Autodesk Inventor part; units mm, degrees
ref_plane "YZ Plane" through (0, 0, 0) normal (1, 0, 0) x (0, 1, 0)
ref_plane "XZ Plane" through (0, 0, 0) normal (0, 1, 0) x (-1, 0, 0)
ref_plane "XY Plane" through (0, 0, 0) normal (0, 0, 1) x (1, 0, 0)
sketch "Sketch1" plane through (0, 0, 0) normal (0, 1, 0) x (-1, 0, 0)
  circle A0 centre (0, 0) radius 3.975
  circle A1 centre (0, 0) radius 5.965
  dimension "d0" = 7.95
  dimension "d1" = 11.93
extrude "Extrusion1" add sketch "Sketch1" along normal blind 7
sketch "Sketch2" plane through (0, 7, 0) normal (0, 1, 0) x (1, 0, 0)
  circle A0 centre (0, 0) radius 5.965
  circle A1 centre (0, 0) radius 11
  dimension "d4" = 22
extrude "Extrusion2" add sketch "Sketch2" against normal up to surface (7 mm away)
sketch "Sketch3" plane through (0, 0, 0) normal (0, -1, 0) x (1, 0, 0)
  circle A0 centre (0, 0) radius 5.96
  circle A1 centre (0, 0) radius 9.725
  dimension "d7" = 11.92
  dimension "d8" = 19.45
extrude "Extrusion3" cut sketch "Sketch3" against normal blind 0.25
sketch "Sketch4" plane through (0, 7, 0) normal (0, 1, 0) x (1, 0, 0)
  circle A0 centre (0, 0) radius 5.96
  circle A1 centre (0, 0) radius 9.725
  circle A2 centre (0, 0) radius 5.96
  circle A3 centre (0, 0) radius 9.725
extrude "Extrusion4" cut sketch "Sketch4" against normal blind 0.25
properties part number "bearing_1"
For this review, take the finished solid that the model builds, in its own axes (mm). A direction names the side the tool comes from. Coordinates: 2 decimals unless noted, no trailing zeros. Loops run counter-clockwise (first coordinate to the right, second up) from the corner with the lowest first, then second, coordinate; pieces in that order, holes last. Notation, with made-up numbers: (20, -3.5) - (53, -3.5) arc R21 ccw to (53, 22.5) - close; hole circle Ø2 at (31.25, 71). An arc over 180 degrees is marked (long way). Use a Markdown table: item, result. Add a question column.
Item 1: We need section A-A (z = 0). Give the boundary of the cut face in (x, y) (3 decimals), and give its area (3 significant figures).
Item 2: Tool access review of faces 1 (the face through (-4.5, 0.25, -4.2)), 2 (the face through (1.4, 0, -3.9)): name each direction out of +Z, -Z, +X, -X, +Y, -Y from which nothing blocks a thin tool from reaching the whole face with its end or side.
Item 3: Mouldability with a two-part tool opening along X and no side actions: class faces 3 (the face through (1.4, 7, -3.9)), 4 (the face through (-4.5, 6.75, 4.2)), 5 (the face through (-2.38, 3.55, 10.74)) as pulls with the +X half, pulls with the -X half, needs draft (parallel to the pull), parting line crosses it, or undercut.
Item 4: We need section D-D (z = 8). Give the boundary of the cut face in (x, y).
Item 5: For line 1 (Z direction, x = 0, y = 0.1) (3 decimals); line 2 (Z direction, x = -0.75, y = 3); line 3 (Y direction, x = 2.75, z = 6), list the stretches that pass through material, from the lowest coordinate up.
Item 6: We need section B-B (x = 0). Give the boundary of the cut face in (y, z) (3 decimals).
Item 7: Insertion check: pin 1 Ø1.5 at (x, y) = (8.5, 5) entering from +Z; pin 2 Ø7 at (x, z) = (0, 0) entering from +Y. Each pin has a flat end and moves straight along its axis. Give the tip position at first contact, or say it passes through.
Item 8: We need section C-C (y = 5.25). Give the boundary of the cut face in (x, z) (3 decimals).
Results list:
| question | item | result |
|---|---|---|
| 1 | outline | (-11, 0) - (-9.725, 0) - (-9.725, 0.25) - (-5.96, 0.25) - (-5.96, 0) - (-3.975, 0) - (-3.975, 7) - (-5.96, 7) - (-5.96, 6.75) - (-9.725, 6.75) - (-9.725, 7) - (-11, 7) - close; (3.975, 0) - (5.96, 0) - (5.96, 0.25) - (9.725, 0.25) - (9.725, 0) - (11, 0) - (11, 7) - (9.725, 7) - (9.725, 6.75) - (5.96, 6.75) - (5.96, 7) - (3.975, 7) - close |
| 1 | area | 94.6 mm^2 |
| 2 | face 1 | -Y |
| 2 | face 2 | +Z, -Z, +X, -X, -Y |
| 3 | face 3 | needs draft |
| 3 | face 4 | undercut |
| 3 | face 5 | parting line crosses it |
| 4 | outline | (-7.55, 0) - (-5.53, 0) - (-5.53, 0.25) - (5.53, 0.25) - (5.53, 0) - (7.55, 0) - (7.55, 7) - (5.53, 7) - (5.53, 6.75) - (-5.53, 6.75) - (-5.53, 7) - (-7.55, 7) - close |
| 5 | line 1 | z = -11 to -9.725, -5.96 to -3.975, 3.975 to 5.96, 9.725 to 11 |
| 5 | line 2 | z = -10.97 to -3.9, 3.9 to 10.97 |
| 5 | line 3 | y = 0.25 to 6.75 |
| 6 | outline | (0, -11) - (7, -11) - (7, -9.725) - (6.75, -9.725) - (6.75, -5.96) - (7, -5.96) - (7, -3.975) - (0, -3.975) - (0, -5.96) - (0.25, -5.96) - (0.25, -9.725) - (0, -9.725) - close; (0, 3.975) - (7, 3.975) - (7, 5.96) - (6.75, 5.96) - (6.75, 9.725) - (7, 9.725) - (7, 11) - (0, 11) - (0, 9.725) - (0.25, 9.725) - (0.25, 5.96) - (0, 5.96) - close |
| 7 | pin 1 | stops at z = 7.81 |
| 7 | pin 2 | passes through |
| 8 | outline | circle Ø22 at (0, 0); hole circle Ø7.95 at (0, 0) |
